Check sheet for the modelled part. Datum: model origin and axes. Units: mm. A direction names the side the tool comes from. Round coordinates to 2 decimals unless told otherwise and drop trailing zeros. Order: outer loops, then holes, each group sorted by start corner. A loop starts at its lowest first (then second) coordinate and runs counter-clockwise, first axis right, second up.
```python
from build123d import *

# Parameters (mm, degrees)
SKETCH1_W           = 4.7625
SKETCH1_H           = 1.545684244
BOSS_EXTRUDE1_DEPTH = 1.524


with BuildPart() as part:
    # Sketch1 → Boss-Extrude1 (new body)
    with BuildSketch(Plane.XY):
        with BuildLine():
            Line((0, 15.440411119), (-1.524, 15.440411119))
            Line((-1.524, 15.440411119), (-1.524, 24.435175852))
            Line((-1.524, 24.435175852), (-1.836778674, 24.435175852))
            ThreePointArc((-1.836778674, 24.435175852), (-2.780560258, 24.253326891), (-3.589203495, 23.733818626))
            ThreePointArc((-3.589203495, 23.733818626), (-11.850131673, 18.109761084), (-21.480683494, 15.440411119))
            ThreePointArc((-21.480683494, 15.440411119), (-23.587055129, 14.543073006), (-24.747192379, 12.569219234))
            ThreePointArc((-24.747192379, 12.569219234), (-17.383897912, 13.471716361), (-9.972791779, 13.142911901))
            ThreePointArc((-9.972791779, 13.142911901), (-8.617730977, 11.821371906), (-6.905922332, 11.013678341))
            ThreePointArc((-6.905922332, 11.013678341), (-8.770219675, 10.681853269), (-9.972791779, 9.219139081))
            ThreePointArc((-9.972791779, 9.219139081), (-17.359992079, 8.625773055), (-24.747192379, 9.219139081))
            ThreePointArc((-24.747192379, 9.219139081), (-24.079326319, 7.561664754), (-23.241579524, 5.983233086))
            ThreePointArc((-23.241579524, 5.983233086), (-22.148302871, 4.993292395), (-20.68927527, 4.777712082))
            ThreePointArc((-20.68927527, 4.777712082), (-10.932367406, 4.867164845), (-1.524, 2.281072115))
            Line((-1.524, 2.281072115), (0, 2.281072115))
            ThreePointArc((0, 2.281072115), (3.282961886, -3.471531025), (9.573778774, -5.544187416))
            ThreePointArc((9.573778774, -5.544187416), (10.603851301, -5.306050671), (11.633923828, -5.544187416))
            Line((11.633923828, -5.544187416), (11.633923828, 16.100831607))
            ThreePointArc((11.633923828, 16.100831607), (6.837865982, 21.693085274), (0, 24.435175852))
            Line((0, 24.435175852), (0, 15.440411119))
        make_face()
        with Locations((-8.66775, 14.92904471)):
            Rectangle(SKETCH1_W, SKETCH1_H, mode=Mode.SUBTRACT)
    extrude(amount=BOSS_EXTRUDE1_DEPTH)


solid = part.part
```
Item 1: Sectioned sample at C-C (y = 18.5). Record the cut outline in (x, z), and give its area (3 significant figures).
Answer:
outline: (-11.04, 0) - (-1.52, 0) - (-1.52, 1.52) - (-11.04, 1.52) - close; (0, 0) - (10.13, 0) - (10.13, 1.52) - (0, 1.52) - close
area: 29.9 mm2
Item 2: Access from +Z, -Z, +X, -X, +Y, -Y to the whole of each face (thin tool, end or side, straight path). Record for faces 1 (the flat face through (-3, 10, 1.524)), 2 (the flat face through (-9, 14.156, 1)), 3 (the flat face through (0, 20, 1)).
Answer:
face 1: +Z, +X, -X, +Y, -Y
face 2: +Z, -Z
face 3: +Z, -Z, +Y
Item 3: Release check for a two-part mould opening along X. For faces 4 (the flat face through (11.634, 5, 1)), 5 (the cylindrical face through (-8.64, 11.837, 0.751)), 6 (the flat face through (-1, 2.281, 1)) record: released by +X, released by -X, zero draft, split by the parting line, or undercut.
Answer:
face 4: released by +X
face 5: undercut
face 6: zero draft
Item 4: Sectioned sample at A-A (x = -9.5). Record the cut outline in (y, z), and give its area (3 significant figures).
Answer:
outline: (4.65, 0) - (10.06, 0) - (10.06, 1.52) - (4.65, 1.52) - close; (12.58, 0) - (14.16, 0) - (14.16, 1.52) - (12.58, 1.52) - close; (15.7, 0) - (19.32, 0) - (19.32, 1.52) - (15.7, 1.52) - close
area: 16.2 mm2
Item 5: Go/stop test with flat-tipped pins: P1, Ø0.8, axis at y = 20, z = 1, coming from the -X side; P2, Ø0.8, axis at x = -0.5, z = 1, coming from the +Y side; P3, Ø0.5, axis at y = 15, z = 1, coming from the -X side. Record where each tip stops, or that it passes through.
Answer:
P1: stops at x = -9.03
P2: stops at y = 15.44
P3: stops at x = -23.33
Item 6: Scan lines: line 1 along X through (y, z) = (15, 1.4); line 2 along X through (y, z) = (19, 1); line 3 along Y through (x, z) = (-15.5, 0.65). Record each from-to range of solid material in increasing order.
Answer:
line 1: x = -22.94 to -11.05, -6.29 to 11.63
line 2: x = -10.08 to -1.52, 0 to 9.73
line 3: y = 5.16 to 8.66, 13.51 to 16.69
Item 7: Sectioned sample at D-D (z = 1.1). Record the cut outline in (x, y).
Answer:
outline: (-24.75, 9.22) arc R17.04 ccw to (-23.24, 5.98) arc R2.54 ccw to (-20.69, 4.78) arc R35.29 cw to (-1.52, 2.28) - (0, 2.28) arc R9.23 ccw to (9.57, -5.54) arc R2.35 cw to (11.63, -5.54) - (11.63, 16.1) arc R15.48 ccw to (0, 24.44) - (0, 15.44) - (-1.52, 15.44) - (-1.52, 24.44) - (-1.84, 24.44) arc R2.54 ccw to (-3.59, 23.73) arc R30.67 cw to (-21.48, 15.44) arc R3.66 ccw to (-24.75, 12.57) arc R44.66 cw to (-9.97, 13.14) arc R5.73 ccw to (-6.91, 11.01) arc R2.74 ccw to (-9.97, 9.22) arc R46.28 cw to start; hole (-11.05, 14.16) - (-6.29, 14.16) - (-6.29, 15.7) - (-11.05, 15.7) - close
Item 8: Sectioned sample at B-B (x = -16). Record the cut outline in (y, z).
Answer:
outline: (5.16, 0) - (8.65, 0) - (8.65, 1.52) - (5.16, 1.52) - close; (13.5, 0) - (16.54, 0) - (16.54, 1.52) - (13.5, 1.52) - close
